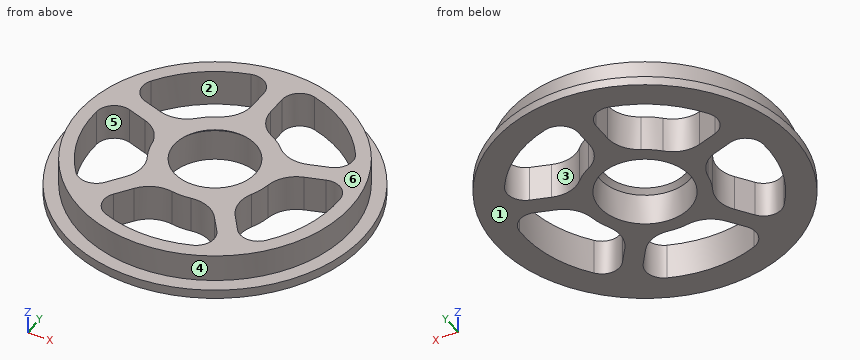
from build123d import *

# Parameters (mm, degrees)
F0_R     = 30
F0_R_2   = 10
F1_DEPTH = 8
F2_R     = 33
F2_R_2   = 30
F3_DEPTH = 2
F4_R     = 10
F4_R_2   = 9
F5_DEPTH = 1
F6_R     = 4
F7_R     = 7
F8_SIZE  = 0.99999


# Not quite as in the source:
# - a fillet or chamfer is up to 0.001 mm smaller than in the source, because OpenCascade refuses the exact size


with BuildPart() as f1:
    # F0 (on Top) → F1 (new body)
    with BuildSketch(Plane.XY):
        Circle(F0_R)
        with BuildLine():
            Line((-14.2085682852, -22.959019737), (-5.9322042833, -11.5675819574))
            ThreePointArc((-5.9322042833, -11.5675819574), (0, -13), (5.9322042833, -11.5675819574))
            Line((5.9322042833, -11.5675819574), (14.2085682852, -22.959019737))
            ThreePointArc((14.2085682852, -22.959019737), (0, -27), (-14.2085682852, -22.959019737))
        make_face(mode=Mode.SUBTRACT)
        with BuildLine():
            Line((-26.2260143945, 6.418424182), (-12.834576136, 2.0672821309))
            ThreePointArc((-12.834576136, 2.0672821309), (-12.3637347118, -4.0172209269), (-9.1682722608, -9.2164409483))
            Line((-9.1682722608, -9.2164409483), (-17.4446362627, -20.6078787278))
            ThreePointArc((-17.4446362627, -20.6078787278), (-25.67852594, -8.3434588481), (-26.2260143945, 6.418424182))
        make_face(mode=Mode.SUBTRACT)
        with BuildLine():
            Line((17.4446362627, -20.6078787278), (9.1682722608, -9.2164409483))
            ThreePointArc((9.1682722608, -9.2164409483), (12.3637347118, -4.0172209269), (12.834576136, 2.0672821309))
            Line((12.834576136, 2.0672821309), (26.2260143945, 6.418424182))
            ThreePointArc((26.2260143945, 6.418424182), (25.67852594, -8.3434588481), (17.4446362627, -20.6078787278))
        make_face(mode=Mode.SUBTRACT)
        with BuildLine():
            Line((-2, 26.9258240357), (-2, 12.8452325787))
            ThreePointArc((-2, 12.8452325787), (-7.6412082798, 10.5172209269), (-11.5985081585, 5.8715081961))
            Line((-11.5985081585, 5.8715081961), (-24.989946417, 10.2226502472))
            ThreePointArc((-24.989946417, 10.2226502472), (-15.8702018119, 21.8434588481), (-2, 26.9258240357))
        make_face(mode=Mode.SUBTRACT)
        Circle(F0_R_2, mode=Mode.SUBTRACT)
        with BuildLine():
            ThreePointArc((11.5985081585, 5.8715081961), (7.6412082798, 10.5172209269), (2, 12.8452325787))
            Line((2, 12.8452325787), (2, 26.9258240357))
            ThreePointArc((2, 26.9258240357), (15.8702018119, 21.8434588481), (24.989946417, 10.2226502472))
            Line((24.989946417, 10.2226502472), (11.5985081585, 5.8715081961))
        make_face(mode=Mode.SUBTRACT)
    extrude(amount=F1_DEPTH)

    # F2 (on face) → F3 (join)
    with BuildSketch(Plane(origin=(0, 0, 0), x_dir=(1, 0, 0), z_dir=(0, 0, -1))):
        Circle(F2_R)
        Circle(F2_R_2, mode=Mode.SUBTRACT)
    extrude(amount=-F3_DEPTH)

    # F4 (on face) → F5 (join)
    with BuildSketch(Plane.XY.offset(8)):
        Circle(F4_R)
        Circle(F4_R_2, mode=Mode.SUBTRACT)
    extrude(amount=-F5_DEPTH)

    # F6
    f6_edges = [f1.edges().sort_by_distance(p)[0] for p in [
        (-26.226014, 6.418424, 4),
        (-24.989946, 10.22265, 4),
        (-17.444636, -20.607879, 4),
        (17.444636, -20.607879, 4),
        (26.226014, 6.418424, 4),
        (-2, 26.925824, 4),
        (-14.208568, -22.95902, 4),
        (14.208568, -22.95902, 4),
        (24.989946, 10.22265, 4),
        (2, 26.925824, 4),
    ]]
    fillet(f6_edges, radius=F6_R)

    # F7
    f7_edges = [f1.edges().sort_by_distance(p)[0] for p in [
        (-12.834576, 2.067282, 4),
        (-9.168272, -9.216441, 4),
        (-5.932204, -11.567582, 4),
        (5.932204, -11.567582, 4),
        (9.168272, -9.216441, 4),
        (12.834576, 2.067282, 4),
        (11.598508, 5.871508, 4),
        (2, 12.845233, 4),
        (-2, 12.845233, 4),
        (-11.598508, 5.871508, 4),
    ]]
    fillet(f7_edges, radius=F7_R)

    # F8 (size 1 in the source; OpenCascade refuses exactly that, so slightly less here)
    f8_edges = [f1.edges().sort_by_distance(p)[0] for p in [
        (-9, 0, 7),
    ]]
    chamfer(f8_edges, length=F8_SIZE)


solid = f1.part
Design review of the part built by this model. Coordinates are the model's own, in mm. Face numbers are marked on the shaded views. A direction names the side the tool comes from. Round coordinates to 2 decimals unless told otherwise and drop trailing zeros. Loops run counter-clockwise (first coordinate to the right, second up) from the corner with the lowest first, then second, coordinate; pieces in that order, holes last. Notation, with made-up numbers: (28, -12) - (38, -12) arc R23 ccw to (38, -1) - close; hole circle Ø6 at (85, 29.5). An arc over 180 degrees is marked (long way). One line per item, written item: value. Start each with the question number.
1) Insertion check: pin 1 Ø2 at (x, z) = (0.5, 5) entering from -Y; pin 2 Ø16 at (x, y) = (1, -3.5) entering from -Z; pin 3 Ø1.5 at (x, z) = (7.5, 3) entering from +Y; pin 4 Ø1 at (x, z) = (-17.5, 5) entering from -Y. Each pin has a flat end and moves straight along its axis. Give the tip position at first contact, or say it passes through.
2) Consider section A-A on x = 0. Give the number of separate pieces and of enclosed holes in the cut face, then the cut area to 3 significant figures.
3) For the marked faces 5 and 6, list the 3-axis set-ups (+Z, -Z, +X, -X, +Y, -Y) from which the entire face can be reached by the end or side of a thin tool; tool diameter is ignored.
4) To check wall thickness, follow L1, parallel to X at y = -3, z = 1; L2, parallel to Y at x = -21.5, z = 7.75; L3, parallel to Y at x = 0, z = 5.75. State the ranges of each line that lie inside material, in increasing order. Write a range as from..to.
5) Consider section B-B on y = -22.5. Give the boundary of the cut face in (x, z).
6) Draft analysis for pull direction X (two halves, no side actions). For the marked faces 1, 2, 3 and 4, state which applies: +X half, -X half, draft (parallel to the pull), parting line (faces both ways), or undercut.
Reported:
1. pin 1: stops at y = -30
1. pin 2: stops at z = 0
1. pin 3: stops at y = 29.23
1. pin 4: stops at y = -24.72
2. separate pieces: 3
2. enclosed holes: 0
2. area: 221 mm^2
3. face 5: +Z, -Z
3. face 6: +Z, +X, -X, +Y, -Y
4. L1: x = -32.86..-26.83, -12.65..-9.54, 9.54..12.65, 26.83..32.86
4. L2: y = -20.92..-16.33, 4.88..9.25, 16.33..20.92
4. L3: y = -30..-27, -13..-10, 10..30
5. outline: (-24.14, 0) - (-12.07, 0) - (-12.07, 8) - (-19.84, 8) - (-19.84, 2) - (-24.14, 2) - close; (12.07, 0) - (24.14, 0) - (24.14, 2) - (19.84, 2) - (19.84, 8) - (12.07, 8) - close
6. face 1: draft
6. face 2: undercut
6. face 3: undercut
6. face 4: parting line
